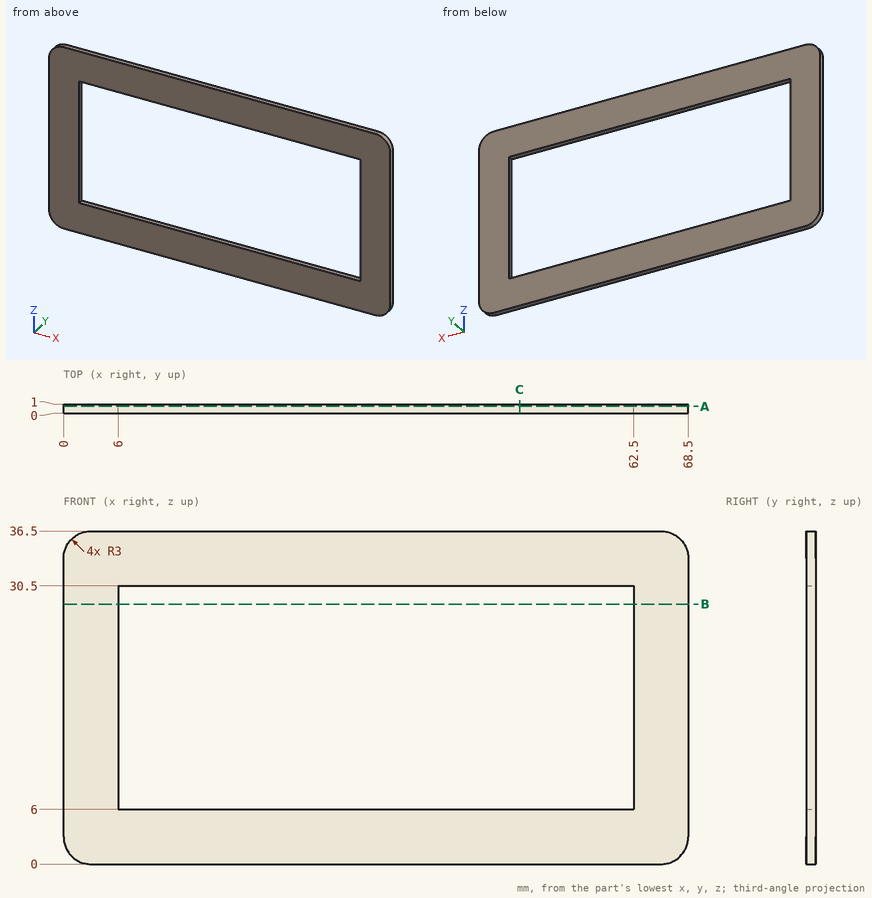
Verification items for this drawing (mm, ordinates from the low corner). Give positions to 0.01 mm unless a question says otherwise; leave off trailing zeros. Order: outer loops, then holes, each group sorted by start corner. A loop starts at its lowest first (then second) coordinate and runs counter-clockwise, first axis right, second up.
1) Cross-section at C-C (x = 50). Record the boundary of the cut face in (y, z), then the cut area to 3 significant figures.
Results are:
outline: (0, 0) - (1, 0) - (1, 6) - (0, 6) - close; (0, 30.5) - (1, 30.5) - (1, 36.5) - (0, 36.5) - close
area: 12.0 mm2
2) Cross-section at A-A (y = 0.75). Record the boundary of the cut face in (x, z).
Results are:
outline: (0, 3) arc R3 ccw to (3, 0) - (65.5, 0) arc R3 ccw to (68.5, 3) - (68.5, 33.5) arc R3 ccw to (65.5, 36.5) - (3, 36.5) arc R3 ccw to (0, 33.5) - close; hole (6, 6) - (62.5, 6) - (62.5, 30.5) - (6, 30.5) - close
3) Gauge pin test, flat end, axial feed: pin 1 (5 mm diameter, centred on x = 9.5, z = 20.5, fed in from -Y). Record the tip position at first contact, or that the pin passes through.
Results are:
pin 1: passes through
4) Material ranges on probe 1 along X at (y, z) = (0.15, 13.5); probe 2 along Z at (x, y) = (51, 0.3), recorded low to high.
Results are:
probe 1: x = 0 to 6, 62.5 to 68.5
probe 2: z = 0 to 6, 30.5 to 36.5
5) Cross-section at B-B (z = 28.5). Record the boundary of the cut face in (x, y).
Results are:
outline: (0, 0) - (6, 0) - (6, 1) - (0, 1) - close; (62.5, 0) - (68.5, 0) - (68.5, 1) - (62.5, 1) - close
